Input: part model. Units: mm. Frame: model coordinates. A direction names the side the tool comes from. Coordinates: 2 decimals unless noted, no trailing zeros. Order: outer loops, then holes, each group sorted by start corner. A loop starts at its lowest first (then second) coordinate and runs counter-clockwise, first axis right, second up. Notation, with made-up numbers: (69.5, -30) - (102.5, -30) arc R11 cw to (102.5, -19) - close; hole circle Ø11 at (85, 23). An arc over 180 degrees is marked (long way). Answer as CSV lines item,"result". Start each with the question number.
Item 1: First-contact query: pin 1 (0.8 mm diameter, centred on y = 4, z = -10, fed in from -X); pin 2 (3 mm diameter, centred on y = 4, z = -31, fed in from -X). Flat tips, straight axial feed; report the tip coordinate or a pass-through.
Item 2: Section A-A (x = -15.5). Output: boundary loops of the cut face in (y, z).
Item 3: Section D-D (z = 46). Output: boundary loops of the cut face in (x, y).
Item 4: Material intervals for line 1 along Z through (x, y) = (79, 2.25); line 2 along Z through (x, y) = (62.5, 5.55); line 3 along X through (y, z) = (0.5, 54), sorted ascending.
Item 5: Draft query along Z for faces 1 (the cylindrical face through (-84.43, 2.96, 59.83)), 2 (the cylindrical face through (-84.33, 2.96, -59.93)), 3 (the flat face through (76.5, 3, 7)), 4 (the flat face through (-86.4, 3, -53)). Return one class per face: +Z half, -Z half, draft (parallel to the pull), parting line (faces both ways), or undercut.
Item 6: Section C-C (y = 2.85). State how many separate pieces and enclosed holes the cut face has, and give its area (3 significant figures).
Item 7: Access query for faces 5 (the cylindrical face through (84.43, 2.96, -59.83)), 6 (the flat face through (61, 3, -7)), 7 (the flat face through (61.23, 3, -17)). Directions: +Z, -Z, +X, -X, +Y, -Y. A direction counts if a zero-diameter tool reaches every point of the face in a straight line with its end or side. Return the directions, or none.
Item 8: Section B-B (z = -45.54). Output: boundary loops of the cut face in (x, y), and give its area (3 significant figures).
from build123d import *

# Parameters (mm, degrees)
SKIZZE1_R                       = 0.0635
SKIZZE1_R_2                     = 1.59999934
SKIZZE1_R_3                     = 1.79999894
AUFSATZ_LINEAR_AUSTRAGEN1_DEPTH = 6


with BuildPart() as part:
    # Skizze1 → Aufsatz-Linear austragen1 (new body)
    with BuildSketch(Plane(origin=(0, 0, 0), x_dir=(1, 0, 0), z_dir=(0, 1, 0))):
        with BuildLine():
            Line((-86.39999891, 50.00000287), (53.43650095, 50.00000287))
            ThreePointArc((53.43650095, 50.00000287), (53.50067303, 50.063499313), (53.563486724, 49.998658786))
            ThreePointArc((53.563486724, 49.998658786), (54.560660834, 49.560663139), (54.998656411, 48.563488998))
            ThreePointArc((54.998656411, 48.563488998), (55.063496933, 48.500675299), (55.000000486, 48.436503224))
            Line((55.000000486, 48.436503224), (54.99999795, 12.500004281))
            ThreePointArc((54.99999795, 12.500004281), (55.292891674, 11.792896174), (55.99999976, 11.5000024))
            ThreePointArc((55.99999976, 11.5000024), (56.707106025, 11.207109395), (56.99999903, 10.50000313))
            Line((56.99999903, 10.50000313), (56.99999903, 8.00000305))
            ThreePointArc((56.99999903, 8.00000305), (57.292892407, 7.292895887), (57.99999957, 7.00000251))
            Line((57.99999957, 7.00000251), (64.24999977, 7.00000251))
            ThreePointArc((64.24999977, 7.00000251), (65.607645667, 6.437647167), (66.17000101, 5.08000127))
            Line((66.17000101, 5.08000127), (66.17000101, -5.07999873))
            ThreePointArc((66.17000101, -5.07999873), (65.607645667, -6.437644627), (64.24999977, -6.99999997))
            Line((64.24999977, -6.99999997), (55.99999849, -6.99999997))
            ThreePointArc((55.99999849, -6.99999997), (55.292892225, -7.292892975), (54.99999922, -7.99999924))
            Line((54.99999922, -7.99999924), (54.99999922, -48.49999952))
            ThreePointArc((54.99999922, -48.49999952), (54.560659527, -49.560659367), (53.49999968, -49.99999906))
            Line((53.49999968, -49.99999906), (-86.40000018, -49.99999906))
            Line((-86.40000018, -49.99999906), (-86.40000018, -54.99999922))
            ThreePointArc((-86.40000018, -54.99999922), (-84.379038194, -59.879033386), (-79.500004221, -61.89999584))
            Line((-79.500004221, -61.89999584), (-5.627e-06, -61.90000346))
            Line((-5.627e-06, -61.90000346), (79.499999141, -61.89999584))
            ThreePointArc((79.499999141, -61.89999584), (84.379034125, -59.879032902), (86.39999637, -54.999997631))
            Line((86.39999637, -54.999997631), (86.39999383, -1.1416e-05))
            Line((86.39999383, -1.1416e-05), (86.39999637, 55.00000049))
            ThreePointArc((86.39999637, 55.00000049), (84.379034012, 59.879035554), (79.499999141, 61.89999838))
            Line((79.499999141, 61.89999838), (0.000118912, 61.900006))
            Line((0.000118912, 61.900006), (-79.50000356, 61.89999838))
            ThreePointArc((-79.50000356, 61.89999838), (-84.379040097, 59.879034549), (-86.40000145, 54.999996985))
            Line((-86.40000145, 54.999996985), (-86.39999891, 50.00000287))
        make_face()
        with Locations(Location((84.99999383, -1.1351e-05, 0), (0, 0, 270))):
            Circle(SKIZZE1_R, mode=Mode.SUBTRACT)
        with BuildLine():
            Line((68.50000016, -8.75000282), (68.50000016, -5.24999966))
            ThreePointArc((68.50000016, -5.24999966), (68.792893537, -4.542892497), (69.5000007, -4.24999912))
            Line((69.5000007, -4.24999912), (75.49999886, -4.24999912))
            ThreePointArc((75.49999886, -4.24999912), (76.207106023, -4.542892497), (76.4999994, -5.24999966))
            Line((76.4999994, -5.24999966), (76.4999994, -8.75000282))
            ThreePointArc((76.4999994, -8.75000282), (76.207106023, -9.457109983), (75.49999886, -9.75000336))
            Line((75.49999886, -9.75000336), (69.5000007, -9.75000336))
            ThreePointArc((69.5000007, -9.75000336), (68.792893537, -9.457109983), (68.50000016, -8.75000282))
        make_face(mode=Mode.SUBTRACT)
        with Locations(Location((-69.9999997, 54.00000122, 0), (0, 0, 270))):
            Circle(SKIZZE1_R_2, mode=Mode.SUBTRACT)
        with BuildLine():
            Line((63.76999946, 23.78650056), (63.76999946, 11.15000056))
            ThreePointArc((63.76999946, 11.15000056), (62.49999946, 9.88000056), (61.22999946, 11.15000056))
            Line((61.22999946, 11.15000056), (61.22999946, 23.85000056))
            ThreePointArc((61.22999946, 23.85000056), (62.46824946, 25.119603623), (63.76841196, 23.913480713))
            ThreePointArc((63.76841196, 23.913480713), (63.833494498, 23.850794372), (63.76999946, 23.78650056))
        make_face(mode=Mode.SUBTRACT)
        with Locations(Location((78.99999948, 40.46000036, 0), (0, 0, 270))):
            Circle(SKIZZE1_R_3, mode=Mode.SUBTRACT)
        with Locations(Location((78.99999948, 45.54000036, 0), (0, 0, 270))):
            Circle(SKIZZE1_R_3, mode=Mode.SUBTRACT)
        with Locations(Location((69.9999997, 54.00000122, 0), (0, 0, 270))):
            Circle(SKIZZE1_R_2, mode=Mode.SUBTRACT)
        with Locations(Location((-69.9999997, -54.00000122, 0), (0, 0, 270))):
            Circle(SKIZZE1_R_2, mode=Mode.SUBTRACT)
        with Locations(Location((69.9999997, -54.00000122, 0), (0, 0, 270))):
            Circle(SKIZZE1_R_2, mode=Mode.SUBTRACT)
    extrude(amount=AUFSATZ_LINEAR_AUSTRAGEN1_DEPTH)


solid = part.part
Determined:
1,pin 1,"stops at x = 57"
1,pin 2,"stops at x = 55"
2,outline,"(0, -61.9) - (6, -61.9) - (6, -50) - (0, -50) - close; (0, 50) - (6, 50) - (6, 61.9) - (0, 61.9) - close"
3,outline,"(55, 0) - (86.4, 0) - (86.4, 6) - (55, 6) - close"
4,line 1,"z = -61.9 to -47.34, -43.74 to -42.26, -38.66 to 61.9"
4,line 2,"z = -61.9 to -25.12, -9.88 to -7, 7 to 61.9"
4,line 3,"x = -86.4 to -71.6, -68.4 to 68.4, 71.6 to 86.4"
5,face 1,"+Z half"
5,face 2,"-Z half"
5,face 3,"undercut"
5,face 4,"draft"
6,separate pieces,"1"
6,enclosed holes,"9"
6,area,"6,920 mm^2"
7,face 5,"-Z, +X, +Y, -Y"
7,face 6,"-X, +Y, -Y"
7,face 7,"+Y, -Y"
8,outline,"(55, 0) - (77.2, 0) - (77.2, 6) - (55, 6) - close; (80.8, 0) - (86.4, 0) - (86.4, 6) - (80.8, 6) - close"
8,area,"167 mm^2"
